```python
from build123d import *

# Parameters (mm, degrees)
F2_R     = 12.065
F3_DEPTH = 12.7
F4_W     = 3.766847
F4_H     = 8.072342
F5_DEPTH = 12.7
F6_W     = 3.766847
F6_H     = 3.006206
F7_DEPTH = 3.048


with BuildPart() as f1:
    # F0 (on Front) → F1 (revolve)
    with BuildSketch(Plane.XZ):
        Polygon((0, 63.5), (0, 0), (15.875, 0), align=None)
    revolve(axis=Axis((0, 0, 31.75), (0, 0, 1)))

    # F2 (on face) → F3 (join)
    with BuildSketch(Plane(origin=(0, 0, 0), x_dir=(1, 0, 0), z_dir=(0, 0, -1))):
        Circle(F2_R)
    extrude(amount=F3_DEPTH)

    # F4 (on Front) → F5 (cut)
    with BuildSketch(Plane.XZ):
        with Locations((-1.883423, -9.887242)):
            Rectangle(F4_W, F4_H)
    extrude(amount=F5_DEPTH, mode=Mode.SUBTRACT)

    # F6 (on face) → F7 (join)
    with BuildSketch(Plane(origin=(0, 0, -12.7), x_dir=(1, 0, 0), z_dir=(0, 0, -1))):
        with Locations((-1.883423, 7.234052)):
            Rectangle(F6_W, F6_H)
    extrude(amount=-F7_DEPTH)


solid = f1.part
```
Input: part model. Units: mm. Frame: model coordinates. A direction names the side the tool comes from. Round coordinates to 2 decimals unless told otherwise and drop trailing zeros. Write each loop counter-clockwise with the first axis right and the second up, starting at its lowest first coordinate (ties: lowest second). Pieces come first, ordered by that corner, then holes. Notation, with made-up numbers: (81, -1.5) -> (105, -1.5) arc R19 cw to (105, 4.5) -> close; hole circle Ø3 at (-35.5, -33.75). An arc over 180 degrees is marked (long way). Answer as CSV lines item,"result".
1. Ray query, L1, parallel to X at y = 7, z = 13.5; L2, parallel to X at y = -5.5, z = 17; L3, parallel to Y at x = 4.5, z = 8 (3 decimals). Return the intervals inside material, ascending. Write a range as [from, to].
Geometry says:
L1,"x = [-10.36, 10.36]"
L2,"x = [-10.24, 10.24]"
L3,"y = [-13.125, 13.125]"
2. Section B-B (z = 13). Return the cut outline in (x, y) (3 decimals).
Geometry says:
outline,"circle Ø25.25 at (0, 0)"
3. Contact query for flat-ended pins moving along their axis: P1, Ø1.5, axis at x = 7, z = 25.5, coming from the -Y side; P2, Ø5.5, axis at y = -8.5, z = -10.5, coming from the -X side; P3, Ø2, axis at y = -3, z = -10, coming from the +X side. Output: stop coordinate, or through.
Geometry says:
P1,"stops at y = -7.2"
P2,"stops at x = -10.61"
P3,"stops at x = 11.9"
4. Reachability of faces 1 (the flat face through (-2, -5.731, -11)), 2 (the flat face through (-2, -6, -5.851)), 3 (the flat face through (0, -6, -9)) from +Z, -Z, +X, -X, +Y, -Y: full face, straight path, thin tool, end or side. Return the list, or none.
Geometry says:
face 1,"-Z"
face 2,"-Y"
face 3,"none"
5. Mould query, pull axis Z, two halves, no side actions, for faces 4 (the flat face through (0, 3, -12.7)), 5 (the flat face through (-2, -8.737, -11)), 6 (the flat face through (-2, -7, -9.652)). Classes: +Z half, -Z half, draft (parallel to the pull), parting line (faces both ways), or undercut.
Geometry says:
face 4,"-Z half"
face 5,"draft"
face 6,"undercut"
6. Section A-A (z = 32.5). Return the cut outline in (x, y).
Geometry says:
outline,"circle Ø15.5 at (0, 0)"
